from build123d import *

# Parameters (mm, degrees)
SKETCH1_W           = 10
SKETCH1_H           = 2
BOSS_EXTRUDE1_DEPTH = 4
SKETCH2_W           = 7.52
SKETCH2_H           = 2.89
CUT_EXTRUDE1_DEPTH  = 1
FILLET1_R           = 0.5
FILLET2_R           = 0.5
SKETCH5_W           = 1.13
SKETCH5_H           = 0.562
CUT_EXTRUDE3_DEPTH  = 0.54
CUT_EXTRUDE8_DEPTH  = 0.25
FILLET4_R           = 0.5


with BuildPart() as part:
    # Sketch1 → Boss-Extrude1 (new body)
    with BuildSketch(Plane.XY):
        with Locations((5, -1)):
            Rectangle(SKETCH1_W, SKETCH1_H)
    extrude(amount=-BOSS_EXTRUDE1_DEPTH)

    # Sketch2 → Cut-Extrude1 (cut)
    with BuildSketch(Plane(origin=(0, 0, 0), x_dir=(1, 0, 0), z_dir=(0, 1, 0))):
        with Locations((5, 2)):
            Rectangle(SKETCH2_W, SKETCH2_H)
    extrude(amount=-CUT_EXTRUDE1_DEPTH, mode=Mode.SUBTRACT)

    # Fillet1
    fillet1_edges = [part.edges().sort_by_distance(p)[0] for p in [
        (10, -1, -4),
        (0, -1, -4),
        (10, -1, 0),
        (0, -1, 0),
    ]]
    fillet(fillet1_edges, radius=FILLET1_R)

    # Fillet2
    fillet2_edges = [part.edges().sort_by_distance(p)[0] for p in [
        (8.76, -0.5, -3.445),
        (8.76, -0.5, -0.555),
        (1.24, -0.5, -0.555),
        (1.24, -0.5, -3.445),
    ]]
    fillet(fillet2_edges, radius=FILLET2_R)

    # Sketch5 → Cut-Extrude3 (cut)
    with BuildSketch(Plane(origin=(0, -1, 0), x_dir=(1, 0, 0), z_dir=(0, 1, 0))):
        with Locations((2.885, 3.164)):
            Rectangle(SKETCH5_W, SKETCH5_H)
        with Locations((7.115, 3.164)):
            Rectangle(SKETCH5_W, SKETCH5_H)
        with Locations((7.115, 0.836)):
            Rectangle(SKETCH5_W, SKETCH5_H)
        with Locations((2.885, 0.836)):
            Rectangle(SKETCH5_W, SKETCH5_H)
    extrude(amount=-CUT_EXTRUDE3_DEPTH, mode=Mode.SUBTRACT)

    # Sketch9 → Cut-Extrude8 (cut)
    with BuildSketch(Plane(origin=(0, 0, 0), x_dir=(1, 0, 0), z_dir=(0, 1, 0))):
        with BuildLine():
            Line((9.9, 0.5), (9.9, 3.5))
            ThreePointArc((9.9, 3.5), (9.782842712, 3.782842712), (9.5, 3.9))
            Line((9.5, 3.9), (0.5, 3.9))
            ThreePointArc((0.5, 3.9), (0.217157288, 3.782842712), (0.1, 3.5))
            Line((0.1, 3.5), (0.1, 0.5))
            ThreePointArc((0.1, 0.5), (0.217157288, 0.217157288), (0.5, 0.1))
            Line((0.5, 0.1), (9.5, 0.1))
            ThreePointArc((9.5, 0.1), (9.782842712, 0.217157288), (9.9, 0.5))
        make_face()
        with BuildLine():
            Line((0.5, 0.2), (9.5, 0.2))
            ThreePointArc((9.5, 0.2), (9.712132034, 0.287867966), (9.8, 0.5))
            Line((9.8, 0.5), (9.8, 3.5))
            ThreePointArc((9.8, 3.5), (9.712132034, 3.712132034), (9.5, 3.8))
            Line((9.5, 3.8), (0.5, 3.8))
            ThreePointArc((0.5, 3.8), (0.287867966, 3.712132034), (0.2, 3.5))
            Line((0.2, 3.5), (0.2, 0.5))
            ThreePointArc((0.2, 0.5), (0.287867966, 0.287867966), (0.5, 0.2))
        make_face(mode=Mode.SUBTRACT)
    extrude(amount=-CUT_EXTRUDE8_DEPTH, mode=Mode.SUBTRACT)

    # Fillet4
    fillet4_edges = [part.edges().sort_by_distance(p)[0] for p in [
        (2.32, -1.54, -3.164),
        (3.45, -1.54, -3.164),
        (2.32, -1.54, -0.836),
        (3.45, -1.54, -0.836),
        (6.55, -1.54, -0.836),
        (7.68, -1.54, -0.836),
        (6.55, -1.54, -3.164),
        (7.68, -1.54, -3.164),
    ]]
    fillet(fillet4_edges, radius=FILLET4_R)


solid = part.part
Part model, mm, in its own coordinate system. A direction names the side the tool comes from. Round coordinates to 2 decimals unless told otherwise and drop trailing zeros. Write each loop counter-clockwise with the first axis right and the second up, starting at its lowest first coordinate (ties: lowest second). Pieces come first, ordered by that corner, then holes. Notation, with made-up numbers: (48.5, 49.5) - (62.5, 49.5) arc R21 cw to (62.5, 86.5) - close; hole circle Ø1 at (61, 23). An arc over 180 degrees is marked (long way). Use CSV: the item, a comma, the result in double quotes.
Item 1: Wall check: L1, parallel to Z at x = 2.5, y = -1.25 (3 decimals); L2, parallel to Z at x = 2, y = -0.4 (3 decimals); L3, parallel to X at y = -0.9, z = -2.2. Give the ranges that are in metal, low to high.
Results list:
L1,"z = -4 to -3.445, -2.883 to -1.117, -0.555 to 0"
L2,"z = -4 to -3.445, -0.555 to 0"
L3,"x = 0 to 1.24, 8.76 to 10"
Item 2: Tool access for faces 1 (the flat face through (5, -1, 0)), 2 (the flat face through (1.24, -0.5, -2)): list every direction of +Z, -Z, +X, -X, +Y, -Y with a clear straight run to the whole face (end or side of a thin tool).
Results list:
face 1,"+Z, +X, -X, +Y, -Y"
face 2,"+Y"
Item 3: Slice it at A-A, the plane y = -0.6. Write the cut outline in (x, z) (3 decimals).
Results list:
outline,"(0, -3.5) arc R0.5 ccw to (0.5, -4) - (9.5, -4) arc R0.5 ccw to (10, -3.5) - (10, -0.5) arc R0.5 ccw to (9.5, 0) - (0.5, 0) arc R0.5 ccw to (0, -0.5) - close; hole (1.24, -2.945) arc R0.5 ccw to (1.74, -3.445) - (8.26, -3.445) arc R0.5 ccw to (8.76, -2.945) - (8.76, -1.055) arc R0.5 ccw to (8.26, -0.555) - (1.74, -0.555) arc R0.5 ccw to (1.24, -1.055) - close"
Item 4: Pull direction Z, two halves, no side cores. Call faces 3 (the flat face through (4.9, 0, -3.6)), 4 (the flat face through (5, -1, -4)), 5 (the flat face through (5, -1, -2)): pulls with the +Z half, pulls with the -Z half, needs draft (parallel to the pull), parting line crosses it, or undercut.
Results list:
face 3,"needs draft"
face 4,"pulls with the -Z half"
face 5,"undercut"
Item 5: Slice it at D-D, the plane y = -1.3. Write the cut outline in (x, z) (3 decimals), then the cut area to 3 significant figures.
Results list:
outline,"(0, -3.5) arc R0.5 ccw to (0.5, -4) - (9.5, -4) arc R0.5 ccw to (10, -3.5) - (10, -0.5) arc R0.5 ccw to (9.5, 0) - (0.5, 0) arc R0.5 ccw to (0, -0.5) - close; hole (2.393, -3.445) - (3.377, -3.445) - (3.377, -2.883) - (2.393, -2.883) - close; hole (2.393, -1.117) - (3.377, -1.117) - (3.377, -0.555) - (2.393, -0.555) - close; hole (6.623, -3.445) - (7.607, -3.445) - (7.607, -2.883) - (6.623, -2.883) - close; hole (6.623, -1.117) - (7.607, -1.117) - (7.607, -0.555) - (6.623, -0.555) - close"
area,"37.6 mm²"
Item 6: Slice it at B-B, the plane x = 5.25. Write the cut outline in (y, z) (3 decimals).
Results list:
outline,"(-2, -4) - (0, -4) - (0, -3.9) - (-0.25, -3.9) - (-0.25, -3.8) - (0, -3.8) - (0, -3.445) - (-1, -3.445) - (-1, -0.555) - (0, -0.555) - (0, -0.2) - (-0.25, -0.2) - (-0.25, -0.1) - (0, -0.1) - (0, 0) - (-2, 0) - close"
Item 7: Slice it at C-C, the plane z = -2.5. Write the cut outline in (x, y), then the cut area to 3 significant figures.
Results list:
outline,"(0, -2) - (10, -2) - (10, 0) - (9.9, 0) - (9.9, -0.25) - (9.8, -0.25) - (9.8, 0) - (8.76, 0) - (8.76, -1) - (1.24, -1) - (1.24, 0) - (0.2, 0) - (0.2, -0.25) - (0.1, -0.25) - (0.1, 0) - (0, 0) - close"
area,"12.4 mm²"
